Autodesk Inventor part; units mm, degrees
ref_plane "YZ Plane" through (0, 0, 0) normal (1, 0, 0) x (0, 1, 0)
ref_plane "XZ Plane" through (0, 0, 0) normal (0, 1, 0) x (-1, 0, 0)
ref_plane "XY Plane" through (0, 0, 0) normal (0, 0, 1) x (1, 0, 0)
sketch "Sketch1" plane through (0, 0, 0) normal (0, 0, 1) x (1, 0, 0)
  arc A0 (69, -46.7929) -> (69.7605, -47) centre (69, -48.2929) ccw
  line L0 (72, -47) -> (69.7605, -47)
  line L1 (72, -72) -> (72, -47)
  line L2 (47, -72) -> (72, -72)
  line L3 (47, -69) -> (47, -72)
  line L4 (22, -69) -> (33, -69)
  line L5 (22, -72) -> (22, -69)
  line L6 (-3, -72) -> (22, -72)
  line L7 (-3, -47) -> (-3, -72)
  line L8 (0, -47) -> (-3, -47)
  line L9 (0, -22) -> (0, -33)
  line L10 (-3, -22) -> (0, -22)
  line L11 (-3, 3) -> (-3, -8.5818)
  line L12 (22, 3) -> (-3, 3)
  line L13 (22, 0) -> (22, 3)
  line L14 (47, 0) -> (36, 0)
  line L15 (47, 3) -> (47, 0)
  line L16 (72, 3) -> (47, 3)
  line L17 (72, -22) -> (72, -9.5)
  line L18 (69, -22) -> (72, -22)
  line L19 (69, -46.7929) -> (69, -36)
  circle A1 centre (17, -3.5) radius 1.5
  circle A2 centre (69, -16.7071) radius 1.5
  circle A3 centre (20, -50.5) radius 1.5
  line L20 (69.7605, -47) -> (69, -47)
  line L21 (69, -47) -> (69, -46.7929)
  line L22 (0, -36) -> (0, -47)
  line L23 (33, 0) -> (22, 0)
  line L24 (69, -33) -> (69, -22)
  line L25 (36, -69) -> (47, -69)
  line L26 (-3, -8.5818) -> (-3, -22)
  circle A4 centre (-1.5, -8.5818) radius 1.5
  line L27 (72, -9.5) -> (72, 3)
  circle A5 centre (70.5, -9.5) radius 1.5
  line L28 (36, -69) -> (36, -62.65)
  line L29 (36, -62.65) -> (38, -62.65)
  line L30 (38, -62.65) -> (38, -60.15)
  line L31 (38, -60.15) -> (36, -60.15)
  line L32 (36, -60.15) -> (36, -56.3)
  line L33 (36, -56.3) -> (33, -56.3)
  line L34 (33, -56.3) -> (33, -60.15)
  line L35 (33, -60.15) -> (31, -60.15)
  line L36 (31, -60.15) -> (31, -62.65)
  line L37 (31, -62.65) -> (33, -62.65)
  line L38 (33, -62.65) -> (33, -69)
  line L39 (0, -36) -> (6.35, -36)
  line L40 (6.35, -36) -> (6.35, -38)
  line L41 (6.35, -38) -> (8.85, -38)
  line L42 (8.85, -38) -> (8.85, -36)
  line L43 (8.85, -36) -> (12.7, -36)
  line L44 (12.7, -36) -> (12.7, -33)
  line L45 (12.7, -33) -> (8.85, -33)
  line L46 (8.85, -33) -> (8.85, -31)
  line L47 (8.85, -31) -> (6.35, -31)
  line L48 (6.35, -31) -> (6.35, -33)
  line L49 (6.35, -33) -> (0, -33)
  line L50 (33, 0) -> (33, -6.35)
  line L51 (33, -6.35) -> (31, -6.35)
  line L52 (31, -6.35) -> (31, -8.85)
  line L53 (31, -8.85) -> (33, -8.85)
  line L54 (33, -8.85) -> (33, -12.7)
  line L55 (33, -12.7) -> (36, -12.7)
  line L56 (36, -12.7) -> (36, -8.85)
  line L57 (36, -8.85) -> (38, -8.85)
  line L58 (38, -8.85) -> (38, -6.35)
  line L59 (38, -6.35) -> (36, -6.35)
  line L60 (36, -6.35) -> (36, 0)
  line L61 (69, -33) -> (62.65, -33)
  line L62 (62.65, -33) -> (62.65, -31)
  line L63 (62.65, -31) -> (60.15, -31)
  line L64 (60.15, -31) -> (60.15, -33)
  line L65 (60.15, -33) -> (56.3, -33)
  line L66 (56.3, -33) -> (56.3, -36)
  line L67 (56.3, -36) -> (60.15, -36)
  line L68 (60.15, -36) -> (60.15, -38)
  line L69 (60.15, -38) -> (62.65, -38)
  line L70 (62.65, -38) -> (62.65, -36)
  line L71 (62.65, -36) -> (69, -36)
  point P0 (0, 0)
extrude "Extrusion1" add sketch "Sketch1" along normal blind 3 contours L21 L20 A0 | A5 | A4 | A0 L0 L1 L2 L3 L25 L28 L29 L30 L31 L32 L33 L34 L35 L36 L37 L38 L4 L5 L6 L7 L8 L22 L39 L40 L41 L42 L43 L44 L45 L46 L47 L48 L49 L9 L10 L26 L11 L12 L13 L23 L50 L51 L52 L53 L54 L55 L56 L57 L58 L59 L60 L14 L15 L16 L27 L17 L18 L24 L61 L62 L63 L64 L65 L66 L67 L68 L69 L70 L71 L19 | A1 | A2 | A3
sketch "Sketch2" plane through (0, 0, 3) normal (0, 0, 1) x (1, 0, 0)
  circle A0 centre (16, -15.05) radius 1.5
  circle A1 centre (53.3, -15.05) radius 1.5
  circle A2 centre (16, -52.35) radius 1.5
  circle A3 centre (53.3, -52.35) radius 1.5
  point P0 (0, 0)
extrude "Extrusion2" cut sketch "Sketch2" against normal blind 3
sketch "Sketch3" plane through (0, 0, 3) normal (0, 0, 1) x (1, 0, 0)
  line L0 (22, 3) -> (-3, 3)
  circle A0 centre (16, -52.35) radius 1.5
  circle A1 centre (16, -15.05) radius 1.5
  circle A2 centre (53.3, -15.05) radius 1.5
  circle A3 centre (53.3, -52.35) radius 1.5
  line L1 (72, -47) -> (69, -47)
  line L2 (69, -47) -> (69, -36)
  line L3 (69, -22) -> (72, -22)
  line L4 (72, -22) -> (72, 3)
  line L5 (72, 3) -> (47, 3)
  line L6 (47, 3) -> (47, 0)
  line L7 (47, 0) -> (36, 0)
  line L8 (22, 0) -> (22, 3)
  line L9 (22, 3) -> (-3, 3)
  line L10 (-3, 3) -> (-3, -22)
  line L11 (-3, -22) -> (0, -22)
  line L12 (0, -22) -> (0, -33)
  line L13 (0, -47) -> (-3, -47)
  line L14 (-3, -47) -> (-3, -72)
  line L15 (-3, -72) -> (22, -72)
  line L16 (22, -72) -> (22, -69)
  line L17 (22, -69) -> (33, -69)
  line L18 (47, -69) -> (47, -72)
  line L19 (47, -72) -> (72, -72)
  line L20 (72, -72) -> (72, -47)
  line L21 (47, 0) -> (22, 0)
  line L22 (34.5, 0) -> (34.5, -12.7)
  line L23 (34.5, -6.35) -> (31, -6.35)
  line L24 (31, -6.35) -> (31, -8.85)
  line L25 (31, -8.85) -> (38, -8.85)
  line L26 (38, -8.85) -> (38, -6.35)
  line L27 (38, -6.35) -> (34.5, -6.35)
  line L28 (34.5, -12.7) -> (36, -12.7)
  line L29 (36, -12.7) -> (36, 0)
  line L30 (34.5, -12.7) -> (33, -12.7)
  line L31 (33, -12.7) -> (33, 0)
  line L32 (33, 0) -> (36, 0)
  line L33 (0, -22) -> (0, -47)
  line L34 (0, -34.5) -> (12.7, -34.5)
  line L35 (6.35, -34.5) -> (6.35, -31)
  line L36 (6.35, -31) -> (8.85, -31)
  line L37 (8.85, -31) -> (8.85, -38)
  line L38 (8.85, -38) -> (6.35, -38)
  line L39 (6.35, -38) -> (6.35, -34.5)
  line L40 (12.7, -34.5) -> (12.7, -36)
  line L41 (12.7, -36) -> (12.7, -33)
  line L42 (12.7, -33) -> (0, -33)
  line L43 (0, -36) -> (0, -33)
  line L44 (0, -36) -> (12.7, -36)
  line L45 (69, -34.5) -> (56.3, -34.5)
  line L46 (62.65, -34.5) -> (62.65, -31)
  line L47 (62.65, -31) -> (60.15, -31)
  line L48 (60.15, -31) -> (60.15, -38)
  line L49 (60.15, -38) -> (62.65, -38)
  line L50 (56.3, -34.5) -> (56.3, -36)
  line L51 (56.3, -36) -> (56.3, -33)
  line L52 (56.3, -33) -> (69, -33)
  line L53 (69, -36) -> (69, -33)
  line L54 (69, -36) -> (56.3, -36)
  line L55 (47, -69) -> (22, -69)
  line L56 (47, -69) -> (22, -69)
  line L57 (34.5, -69) -> (34.5, -56.3)
  line L58 (34.5, -62.65) -> (31, -62.65)
  line L59 (31, -62.65) -> (31, -60.15)
  line L60 (31, -60.15) -> (38, -60.15)
  line L61 (38, -60.15) -> (38, -62.65)
  line L62 (38, -62.65) -> (34.5, -62.65)
  line L63 (34.5, -56.3) -> (36, -56.3)
  line L64 (36, -56.3) -> (36, -69)
  line L65 (34.5, -56.3) -> (33, -56.3)
  line L66 (33, -56.3) -> (33, -69)
  line L67 (33, -69) -> (36, -69)
  line L68 (0, -33) -> (12.7, -33)
  line L69 (12.7, -33) -> (12.7, -36)
  line L70 (12.7, -36) -> (0, -36)
  line L71 (0, -36) -> (0, -33)
  line L72 (33, 0) -> (36, 0)
  line L73 (36, 0) -> (36, -12.7)
  line L74 (36, -12.7) -> (33, -12.7)
  line L75 (33, -12.7) -> (33, 0)
  line L76 (56.3, -33) -> (69, -33)
  line L77 (69, -33) -> (69, -36)
  line L78 (69, -36) -> (56.3, -36)
  line L79 (56.3, -36) -> (56.3, -33)
  line L80 (33, -56.3) -> (36, -56.3)
  line L81 (36, -56.3) -> (36, -69)
  line L82 (36, -69) -> (33, -69)
  line L83 (33, -69) -> (33, -56.3)
  line L84 (60.15, -38) -> (62.65, -38)
  line L85 (62.65, -38) -> (62.65, -31)
  line L86 (62.65, -31) -> (60.15, -31)
  line L87 (60.15, -31) -> (60.15, -38)
  line L88 (69, -33) -> (69, -22)
  line L89 (33, 0) -> (22, 0)
  line L90 (0, -36) -> (0, -47)
  line L91 (36, -69) -> (47, -69)
  line L92 (69, -36) -> (62.65, -36)
  line L93 (62.65, -36) -> (62.65, -38)
  line L94 (62.65, -38) -> (60.15, -38)
  line L95 (60.15, -38) -> (60.15, -36)
  line L96 (60.15, -36) -> (56.3, -36)
  line L97 (56.3, -36) -> (56.3, -33)
  line L98 (56.3, -33) -> (60.15, -33)
  line L99 (60.15, -33) -> (60.15, -31)
  line L100 (60.15, -31) -> (62.65, -31)
  line L101 (62.65, -31) -> (62.65, -33)
  line L102 (62.65, -33) -> (69, -33)
  line L103 (36, 0) -> (36, -6.35)
  line L104 (36, -6.35) -> (38, -6.35)
  line L105 (38, -6.35) -> (38, -8.85)
  line L106 (38, -8.85) -> (36, -8.85)
  line L107 (36, -8.85) -> (36, -12.7)
  line L108 (36, -12.7) -> (33, -12.7)
  line L109 (33, -12.7) -> (33, -8.85)
  line L110 (33, -8.85) -> (31, -8.85)
  line L111 (31, -8.85) -> (31, -6.35)
  line L112 (31, -6.35) -> (33, -6.35)
  line L113 (33, -6.35) -> (33, 0)
  line L114 (0, -33) -> (6.35, -33)
  line L115 (6.35, -33) -> (6.35, -31)
  line L116 (6.35, -31) -> (8.85, -31)
  line L117 (8.85, -31) -> (8.85, -33)
  line L118 (8.85, -33) -> (12.7, -33)
  line L119 (12.7, -33) -> (12.7, -36)
  line L120 (12.7, -36) -> (8.85, -36)
  line L121 (8.85, -36) -> (8.85, -38)
  line L122 (8.85, -38) -> (6.35, -38)
  line L123 (6.35, -38) -> (6.35, -36)
  line L124 (6.35, -36) -> (0, -36)
  line L125 (33, -69) -> (33, -62.65)
  line L126 (33, -62.65) -> (31, -62.65)
  line L127 (31, -62.65) -> (31, -60.15)
  line L128 (31, -60.15) -> (33, -60.15)
  line L129 (33, -60.15) -> (33, -56.3)
  line L130 (33, -56.3) -> (36, -56.3)
  line L131 (36, -56.3) -> (36, -60.15)
  line L132 (36, -60.15) -> (38, -60.15)
  line L133 (38, -60.15) -> (38, -62.65)
  line L134 (38, -62.65) -> (36, -62.65)
  line L135 (36, -62.65) -> (36, -69)
  point P0 (0, 0)
  dimension "d4" = 12.7
  dimension "d5" = 3.5
  dimension "d6" = 2.5
  dimension "d7" = 7
  dimension "d8" = 1.5
  dimension "d9" = 1.5
  dimension "d10" = 12.7
  dimension "d11" = 3.5
  dimension "d12" = 2.5
  dimension "d13" = 7
  dimension "d14" = 1.5
  dimension "d15" = 3
extrude "Extrusion3" cut sketch "Sketch3" against normal blind 25.4 contours L21 L22 L23 L31 | L21 L29 L27 L22 | L31 L25 L24 L23 | L23 L22 L25 L31 | L42 L35 L34 L33 | L27 L29 L25 L22 | L25 L22 L30 L31 | L34 L39 L44 L33 | L42 L37 L34 L35 | L35 L36 L37 L42 | L27 L26 L25 L29 | L25 L29 L28 L22 | L34 L37 L44 L39 | L42 L41 L34 L37 | L44 L37 L38 L39 | L34 L40 L44 L37 | L53 L45 L46 L52 | L52 L48 L47 L46 | L46 L45 L48 L52 | L53 L54 L85 L45 | L66 L58 L57 L55 | L85 L54 L48 L45 | L48 L45 L51 L52 | L57 L62 L64 L55 | L66 L60 L57 L58 | L58 L59 L60 L66 | L48 L54 L50 L45 | L85 L49 L48 L54 | L57 L60 L64 L62 | L66 L65 L57 L60 | L64 L60 L61 L62 | L57 L63 L64 L60
sketch "Sketch4" plane through (0, 0, 3) normal (0, 0, 1) x (1, 0, 0)
  line L0 (-3, -11) -> (-3, -8)
  line L1 (-3, 3) -> (-3, -22)
  line L2 (-3, -9.5) -> (-1.5, -9.5)
  line L3 (72, -22) -> (72, 3)
  line L4 (72, -9.5) -> (70.5, -9.5)
  circle A0 centre (70.5, -9.5) radius 1.5
  circle A1 centre (-1.5, -9.5) radius 1.5
  point P0 (0, 0)
  dimension "d18" = 1.5
  dimension "d19" = 1.5
extrude "Extrusion4" cut sketch "Sketch4" against normal blind 25.4
sketch "Sketch5" plane through (72, 3, 3) normal (1, 0, 0) x (0, 0, -1)
  line L0 (0, -12.5) -> (3, -12.5)
  line L1 (3, -12.5) -> (3, 0)
  line L2 (3, 0) -> (0, 0)
  line L3 (0, -12.5) -> (0, 0)
  line L4 (0, -25) -> (0, -12.5)
  line L5 (3, -25) -> (0, -25)
  line L6 (3, -25) -> (3, -12.5)
  point P0 (3, -3)
extrude "Extrusion5" add sketch "Sketch5" along normal blind 0.5
sketch "Sketch6" plane through (-3, 3, 0) normal (-1, 0, 0) x (0, 0, 1)
  line L0 (3, -12.5) -> (0, -12.5)
  line L1 (3, 0) -> (3, -12.5)
  line L2 (0, 0) -> (3, 0)
  line L3 (0, 0) -> (0, -12.5)
  line L4 (0, -12.5) -> (0, -25)
  line L5 (0, -25) -> (3, -25)
  line L6 (3, -12.5) -> (3, -25)
  line L7 (3, -12.5) -> (0, -12.5)
  line L8 (0, -12.5) -> (0, -25)
  line L9 (0, -25) -> (3, -25)
  line L10 (3, -12.5) -> (3, -25)
  line L11 (3, 0) -> (3, -12.5)
  line L12 (0, 0) -> (3, 0)
  line L13 (0, 0) -> (0, -12.5)
  point P0 (0, -3)
extrude "Extrusion6" add sketch "Sketch6" along normal blind 0.5
properties part number "pared ateral 2"
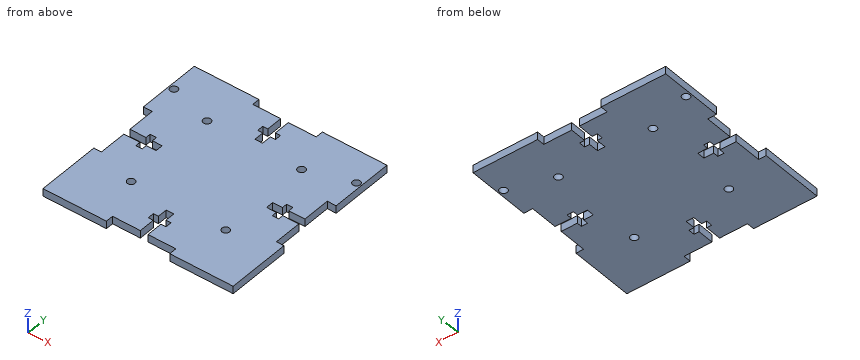
Input: part model. Units: mm. Frame: model coordinates. Give positions to 0.01 mm unless a question says otherwise; leave off trailing zeros. Order: outer loops, then holes, each group sorted by start corner. A loop starts at its lowest first (then second) coordinate and runs counter-clockwise, first axis right, second up. Notation, with made-up numbers: (65.25, 40) - (109.25, 40) arc R32 ccw to (109.25, 78) - close; hole circle Ø11 at (11, 2). An arc over 180 degrees is marked (long way). Write each question's results on one line, items separated by ' | '.
Item 1: Section C-C (z = 1). Give the number of separate pieces and of enclosed holes in the cut face, and give its area (3 significant figures).
A:
separate pieces: 1 | enclosed holes: 6 | area: 5,120 mm^2
Item 2: Material intervals for line 1 along Y through (x, z) = (-1.5, 1.9); line 2 along Y through (x, z) = (53.3, 1.45); line 3 along X through (y, z) = (-15, 0.9), sorted ascending.
A:
line 1: y = -72 to -47, -22 to -11, -8 to 3 | line 2: y = -72 to -53.85, -50.85 to -16.55, -13.55 to 3 | line 3: x = -3.5 to 14.5, 17.5 to 51.8, 54.8 to 72.5
Item 3: Section A-A (x = 70.5). Return loops of the section in (y, z).
A:
outline: (-72, 0) - (-47, 0) - (-47, 3) - (-72, 3) - close; (-22, 0) - (-11, 0) - (-11, 3) - (-22, 3) - close; (-8, 0) - (3, 0) - (3, 3) - (-8, 3) - close
Item 4: Section B-B (y = -15.05). Return loops of the section in (x, z).
A:
outline: (-3.5, 0) - (14.5, 0) - (14.5, 3) - (-3.5, 3) - close; (17.5, 0) - (51.8, 0) - (51.8, 3) - (17.5, 3) - close; (54.8, 0) - (72.5, 0) - (72.5, 3) - (54.8, 3) - close
Item 5: Section D-D (x = 35). Return loops of the section in (y, z), and give its area (3 significant figures).
A:
outline: (-56.3, 0) - (-12.7, 0) - (-12.7, 3) - (-56.3, 3) - close | area: 131 mm^2
Item 6: Contact query for flat-ended pins moving along their axis: pin 1 Ø1.6 at (y, z) = (-32.5, 2) entering from -X; pin 2 Ø1 at (y, z) = (-63, 1) entering from +X; pin 3 Ø0.6 at (x, z) = (32.5, 1) entering from +Y; pin 4 Ø6 at (x, y) = (15.5, -10) entering from -Z. Output: stop coordinate, or through.
A:
pin 1: stops at x = 0 | pin 2: stops at x = 72 | pin 3: stops at y = 0 | pin 4: stops at z = 0
